from build123d import *
from build123d.topology import SkipClean

# Parameters (mm, degrees)
BODY_ANGLE   = 180
INSIDE_ANGLE = 180
LIP_START    = 1.27
SKETCH4_R    = 9.652
SKETCH4_R_2  = 8.89
LIP_DEPTH    = 1.27


with BuildPart() as part:
    # Sketch1 → Body (revolve)
    with BuildSketch(Plane.XY):
        with BuildLine():
            Line((0, 0), (8.89, 0))
            Line((8.89, 0), (8.89, 6.35))
            ThreePointArc((8.89, 6.35), (7.774076836, 9.044076836), (5.08, 10.16))
            Line((5.08, 10.16), (0, 10.16))
            Line((0, 10.16), (0, 0))
        make_face()
    revolve(axis=Axis((0, 0, 0), (0, 1, 0)), revolution_arc=BODY_ANGLE)

    # Sketch2 → Inside (revolve, cut)
    with BuildSketch(Plane.XY):
        with BuildLine():
            Line((0, 0), (8.128, 0))
            Line((8.128, 0), (8.128, 5.842))
            ThreePointArc((8.128, 5.842), (7.235261469, 7.997261469), (5.08, 8.89))
            Line((5.08, 8.89), (0, 8.89))
            Line((0, 8.89), (0, 0))
        make_face()
    revolve(axis=Axis((0, 0, 0), (0, 1, 0)), revolution_arc=INSIDE_ANGLE, mode=Mode.SUBTRACT)

    # Mirror 2: part across face


with BuildPart() as part_1:
    with SkipClean():  # the faces are left unmerged after this step: merging them gives an invalid solid
        add(part.part)
        add(part.part.mirror(Plane(origin=(0, 7.378791693, 0), x_dir=(1, 0, 0), z_dir=(0, 0, 1))))

    # Sketch4 → Lip (add)
    with SkipClean():  # the faces are left unmerged after this step: merging them gives an invalid solid
        with BuildSketch(Plane(origin=(0, 0, 0), x_dir=(1, 0, 0), z_dir=(0, 1, 0)).offset(LIP_START)):
            with Locations(Location((0, 0, 0), (0, 0, 270))):
                Circle(SKETCH4_R)
            with Locations(Location((0, 0, 0), (0, 0, 90))):
                Circle(SKETCH4_R_2, mode=Mode.SUBTRACT)
        extrude(amount=-LIP_DEPTH)


solid = part_1.part
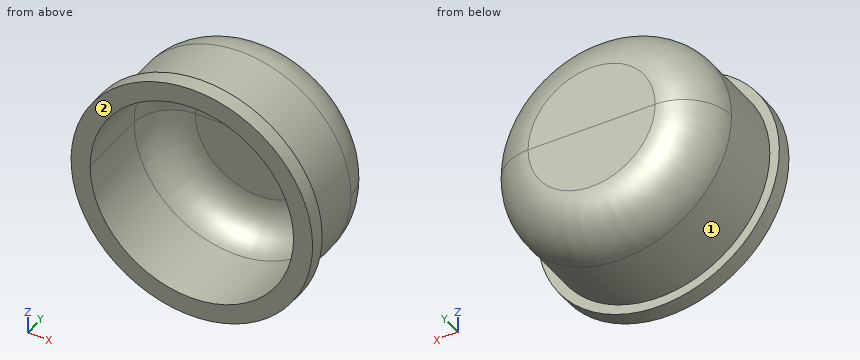
Here's how the part is built. I have some questions about the finished solid (model axes, mm). Face numbers are marked on the shaded views. A direction names the side the tool comes from. Give positions to 0.01 mm unless a question says otherwise; leave off trailing zeros. Loops run counter-clockwise (first coordinate to the right, second up) from the corner with the lowest first, then second, coordinate; pieces in that order, holes last. Notation, with made-up numbers: (57.5, 18) -> (75.5, 18) arc R16 cw to (75.5, 30) -> close; hole circle Ø2 at (-31.75, 77). An arc over 180 degrees is marked (long way). One line per item, written item: value.
Q1. I'm going to push flat-ended pins straight in: pin 1 Ø4 at (x, y) = (2, 2.5) entering from +Z; pin 2 Ø1 at (x, y) = (-7.5, 2.5) entering from -Z; pin 3 Ø5 at (x, y) = (6, 8.5) entering from +Z. Where does each tip first touch, or does it pass through?
Answers follow:
pin 1: z = 9.64
pin 2: z = -5.48
pin 3: z = 7.9
Q2. Suppose I cut it at C-C on y = 5. Please give me the cut outline in (x, z).
Answers follow:
outline: circle Ø17.78 at (0, 0); hole circle Ø16.26 at (0, 0)
Q3. Suppose I cut it at A-A on x = 0. Please give me the cut outline in (y, z).
Answers follow:
outline: (0, -9.65) -> (1.27, -9.65) -> (1.27, -8.89) -> (6.35, -8.89) arc R3.81 ccw to (10.16, -5.08) -> (10.16, 5.08) arc R3.81 ccw to (6.35, 8.89) -> (1.27, 8.89) -> (1.27, 9.65) -> (0, 9.65) -> (0, 8.13) -> (5.84, 8.13) arc R3.05 cw to (8.89, 5.08) -> (8.89, -5.08) arc R3.05 cw to (5.84, -8.13) -> (0, -8.13) -> close
Q4. On a 3-axis mill with a long thin cutter (end or side, diameter ignored), from which of +Z, -Z, +X, -X, +Y, -Y can I reach the whole of each face in a straight line? I mean the marked faces 1 and 2. Say none if no direction works.
Answers follow:
face 1: +Y
face 2: +Z, -Z, +X, -X, -Y
Q5. Suppose I cut it at B-B on y = 1. Please give me the cut outline in (x, z), then the cut area to 3 significant figures.
Answers follow:
outline: circle Ø19.3 at (0, 0); hole circle Ø16.26 at (0, 0)
area: 85.1 mm^2
Q6. If I drill on line 1 along X through (y, z) = (1.5, -0.25); line 2 along X through (y, z) = (0.5, 3.5); line 3 along Z through (x, y) = (6.75, 7), over which ranges is the centre line in solid material (lowest first)?
Answers follow:
line 1: -8.89 to -8.12, 8.12 to 8.89
line 2: -9 to -7.34, 7.34 to 9
line 3: -5.7 to -4.1, 4.1 to 5.7
